from build123d import *
from build123d.topology import SkipClean

# Parameters (mm, degrees)
CHAMFERROD_SIZE   = 0.5
CROSS_DEPTH       = 2.8
CIRPATTERN1_COUNT = 4
FILLET1_R         = 0.3


with BuildPart() as part:
    # Sketch1 → RevolveBase (revolve)
    with BuildSketch(Plane(origin=(0, 0, 0), x_dir=(0, 0, -1), z_dir=(1, 0, 0)), mode=Mode.PRIVATE) as revolvebase_sk:
        Polygon((0, 0), (0, 2.8), (0.35, 2.8), (1.65, 1.5), (6, 1.5), (6, 0), align=None)
    revolve(revolvebase_sk.sketch.rotate(Axis((0, 0, 0), (0, 0, -1)), 90), axis=Axis((0, 0, 0), (0, 0, -1)))

    # ChamferRod
    chamferrod_edges = [part.edges().sort_by_distance(p)[0] for p in [
        (-1.5, 0, -6),
    ]]
    chamfer(chamferrod_edges, length=CHAMFERROD_SIZE)

    # Sketch3 → Cross (cut)
    with BuildSketch(Plane.XY):
        with BuildLine():
            Line((-0.342946789, 0), (0.342946789, 0))
            Line((0.342946789, 0), (0.342946789, 1.357345756))
            ThreePointArc((0.342946789, 1.357345756), (0, 1.4), (-0.342946789, 1.357345756))
            Line((-0.342946789, 1.357345756), (-0.342946789, 0))
        make_face()
    cross = extrude(amount=-CROSS_DEPTH, mode=Mode.SUBTRACT)

    # CirPattern1: Cross ×4 about axis
    cirpattern1_axis = Axis((0, 0, 0), (0, 0, 1))
    for i in range(1, CIRPATTERN1_COUNT):
        add(cross.rotate(cirpattern1_axis, i * 360 / CIRPATTERN1_COUNT), mode=Mode.SUBTRACT)

    # Sketch5 → RevolveRod (revolve)
    with BuildSketch(Plane(origin=(0, 0, 0), x_dir=(0, 0, -1), z_dir=(1, 0, 0)), mode=Mode.PRIVATE) as revolverod_sk:
        Polygon((2.8, 0), (2.8, 1.9), (0, 1.9), (0, 1.4), (1.534352627, 0.635), (1.871988116, 0), align=None)
    revolve(revolverod_sk.sketch.rotate(Axis((0, 0, 0), (0, 0, -1)), 90), axis=Axis((0, 0, 0), (0, 0, -1)))

    # Sketch7 → CutRod (revolve, cut)
    with SkipClean():  # the faces are left unmerged after this step: merging them gives an invalid solid
        with BuildSketch(Plane(origin=(0, 0, 0), x_dir=(0, 0, -1), z_dir=(1, 0, 0)), mode=Mode.PRIVATE) as cutrod_sk:
            Polygon((-21.85, 25), (1.65, 1.5), (2.8, 1.5), (2.8, 25), align=None)
        revolve(cutrod_sk.sketch.rotate(Axis((0, 0, 0), (0, 0, -1)), 90), axis=Axis((0, 0, 0), (0, 0, -1)), mode=Mode.SUBTRACT)

    # Fillet1
    fillet1_edges = [part.edges().sort_by_distance(p)[0] for p in [
        (-1.5, 0, -1.65),
    ]]
    fillet(fillet1_edges, radius=FILLET1_R)


solid = part.part
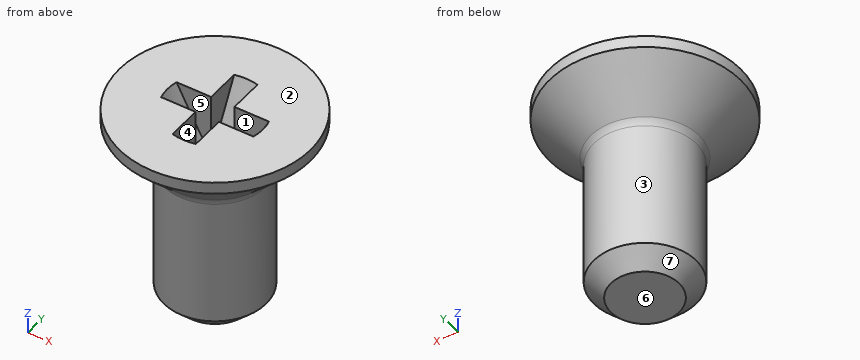
Can you work these out from the model? Positions are in its coordinate system, mm. Face numbers are marked on the shaded views. A direction names the side the tool comes from. Coordinates: 2 decimals unless noted, no trailing zeros. Loops run counter-clockwise (first coordinate to the right, second up) from the corner with the lowest first, then second, coordinate; pieces in that order, holes last. Notation, with made-up numbers: M 54.5,-9.75 L 64.5,-9.75 A17 cw 64.5,11.25 Z; hole C 89.5,86.25 d10. An arc over 180 degrees is marked long. Return JSON: item names as keys, results as strings. Group by question number.
Item 1: Imagine slicing it at B-B (z = -4.65). Please give me the cut outline in (x, y).
Item 2: If I drill on L1, parallel to Y at x = 0.05, z = -4.8; L2, parallel to X at y = 0.3, z = -1.8; L3, parallel to X at y = -1.2, z = -1.9, over which ranges is the centre line in solid material (lowest first)? Write a range as from..to.
Item 3: Thinking about a two-plate mould opening in X: for the marked faces 4, 5, 6 and 7, which applies, released by +X, released by -X, zero draft, split by the parting line, or undercut?
Item 4: I'm going to push flat-ended pins straight in: pin 1 Ø1.1 at (x, z) = (1, -0.5) entering from +Y; pin 2 Ø1.1 at (y, z) = (-1, -0.5) entering from -X; pin 3 Ø1 at (x, z) = (1.5, -4) entering from +Y. Where does each tip first touch, or does it pass through?
Item 5: On a 3-axis mill with a long thin cutter (end or side, diameter ignored), from which of +Z, -Z, +X, -X, +Y, -Y can I reach the whole of each face in a straight line? I mean the marked faces 1, 2 and 3. Say none if no direction works.
Item 6: Imagine slicing it at A-A (z = -0.5). Please give me the cut outline in (x, y).
Verdict:
{
 "1": {"outline": "C 0,0 d3"},
 "2": {"L1": "y = -1.5..1.5", "L2": "x = -1.47..1.47", "L3": "x = -0.9..0.9"},
 "3": {"face 4": "undercut", "face 5": "undercut", "face 6": "zero draft", "face 7": "split by the parting line"},
 "4": {"pin 1": "stops at y = 2.76", "pin 2": "stops at x = -2.76", "pin 3": "stops at y = 1.12"},
 "5": {"face 1": "+Z", "face 2": "+Z, +X, -X, +Y, -Y", "face 3": "-Z"},
 "6": {"outline": "C 0,0 d5.3; hole M -1.1,-0.34 L -0.34,-0.34 L -0.34,-1.1 A1.15 ccw 0.34,-1.1 L 0.34,-0.34 L 1.1,-0.34 A1.15 ccw 1.1,0.34 L 0.34,0.34 L 0.34,1.1 A1.15 ccw -0.34,1.1 L -0.34,0.34 L -1.1,0.34 A1.15 ccw Z"}
}
